Part print with two shaded views. Sizes in mm from the minimum x, y, z corner. Round coordinates to 2 decimals unless told otherwise and drop trailing zeros. Order: outer loops, then holes, each group sorted by start corner. A loop starts at its lowest first (then second) coordinate and runs counter-clockwise, first axis right, second up. Notation, with made-up numbers: (-13, 42.5) -> (28, 42.5) arc R20 cw to (28, 73.5) -> close; hole circle Ø10 at (87, 40.25). An arc over 180 degrees is marked (long way). Use a Markdown table: item, result. Add a question column.
Item 1: Two-plate mould, pull along X, no slides. Class the marked faces 1, 2 and 3: released by +X, released by -X, zero draft, split by the parting line, or undercut.
Item 2: Pin check, flat tips, straight feed: pin 1 (12 mm diameter, centred on x = 50.5, y = 108.5, fed in from +Z); pin 2 (3 mm diameter, centred on x = 17.5, y = 204.5, fed in from -Z); pin 3 (6 mm diameter, centred on x = 13, y = 68, fed in from +Z). Stop position of each tip, or through.
Item 3: Probe L1, parallel to Z at x = 40, y = 4; L2, parallel to Y at x = 7, z = 38.5; L3, parallel to X at y = 80, z = 42. List the from-to ranges inside material, lowest first.
Item 4: Slice it at D-D, the plane z = 58.5. Give the cut face in (x, y).
Item 5: Slice it at C-C, the plane y = 191. Give the cut face in (x, z), plus the area to 3 significant figures.
Item 6: Slice it at B-B, the plane x = 40. Give the cut face in (y, z), plus the area to 4 significant figures.
Item 7: Slice it at A-A, the plane z = 40. Give the cut face in (x, y), plus the area to 4 significant figures.
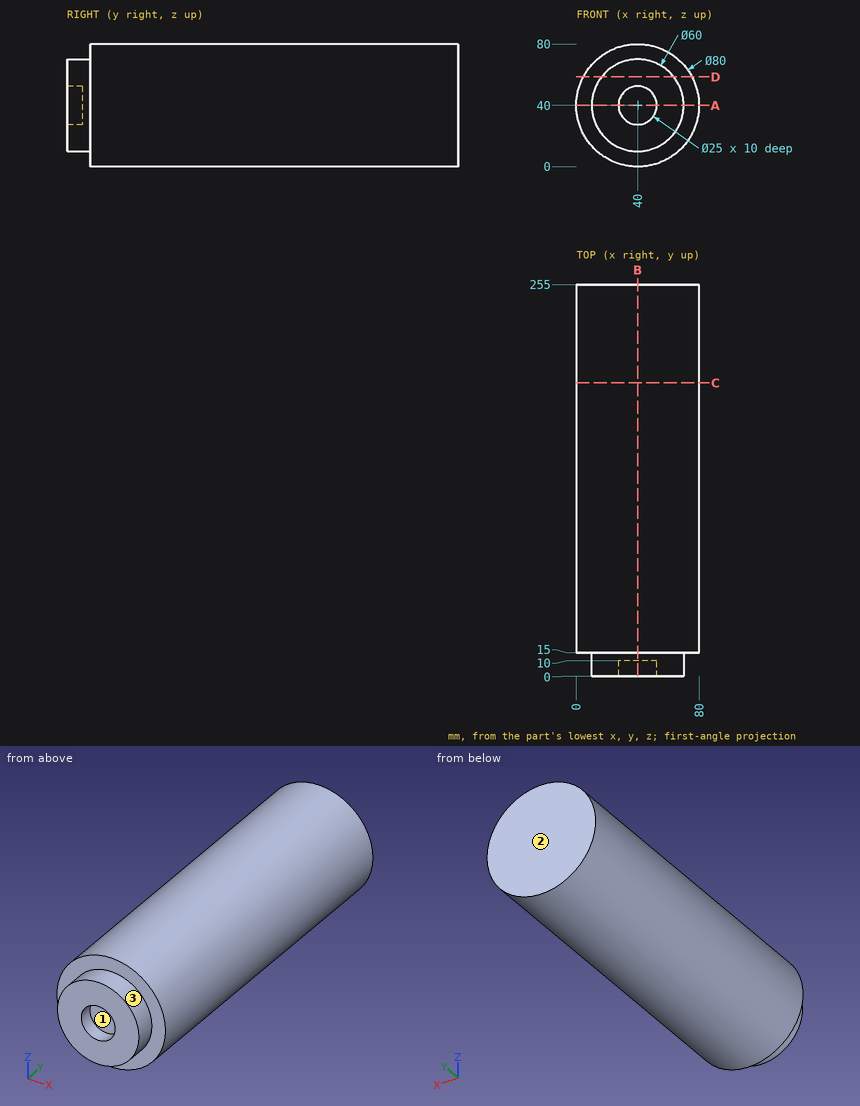
Check sheet entries:
| question | item | result |
|---|---|---|
| 1 | face 1 | undercut |
| 1 | face 2 | zero draft |
| 1 | face 3 | split by the parting line |
| 2 | pin 1 | z = 79.75 |
| 2 | pin 2 | z = 5.96 |
| 2 | pin 3 | z = 72 |
| 3 | L1 | 10 to 27.5, 52.5 to 70 |
| 3 | L2 | 15 to 255 |
| 3 | L3 | 0.05 to 79.95 |
| 4 | outline | (4.54, 15) -> (16.38, 15) -> (16.38, 0) -> (63.62, 0) -> (63.62, 15) -> (75.46, 15) -> (75.46, 255) -> (4.54, 255) -> close |
| 5 | outline | circle Ø80 at (40, 40) |
| 5 | area | 5,030 mm2 |
| 6 | outline | (0, 10) -> (15, 10) -> (15, 0) -> (255, 0) -> (255, 80) -> (15, 80) -> (15, 70) -> (0, 70) -> (0, 52.5) -> (10, 52.5) -> (10, 27.5) -> (0, 27.5) -> close |
| 6 | area | 19,850 mm2 |
| 7 | outline | (0, 15) -> (10, 15) -> (10, 0) -> (27.5, 0) -> (27.5, 10) -> (52.5, 10) -> (52.5, 0) -> (70, 0) -> (70, 15) -> (80, 15) -> (80, 255) -> (0, 255) -> close |
| 7 | area | 19,850 mm2 |
